Here's how the part is built. I have some questions about the finished solid (model axes, mm). A direction names the side the tool comes from. Coordinates: 2 decimals unless noted, no trailing zeros. Write each loop counter-clockwise with the first axis right and the second up, starting at its lowest first coordinate (ties: lowest second). Pieces come first, ordered by that corner, then holes. Notation, with made-up numbers: (0, -17) -> (40, -17) arc R4 cw to (40, -13) -> close; hole circle Ø1 at (-2, 61.25). An arc over 180 degrees is marked (long way). Use a Markdown table: item, result. Add a question column.
```python
from build123d import *

# Parameters (mm, degrees)
SKETCH1_W           = 50
SKETCH1_H           = 50
BOSS_EXTRUDE1_DEPTH = 10
SKETCH2_R           = 17
CUT_EXTRUDE1_DEPTH  = 10
SKETCH3_R           = 4
BOSS_EXTRUDE2_DEPTH = 10


with BuildPart() as part:
    # Sketch1 → Boss-Extrude1 (new body)
    with BuildSketch(Plane.XY):
        Rectangle(SKETCH1_W, SKETCH1_H)
    extrude(amount=BOSS_EXTRUDE1_DEPTH)

    # Sketch2 → Cut-Extrude1 (cut)
    with BuildSketch(Plane.XY.offset(10)):
        Circle(SKETCH2_R)
    extrude(amount=-CUT_EXTRUDE1_DEPTH, mode=Mode.SUBTRACT)

    # Sketch3 → Boss-Extrude2 (add)
    with BuildSketch(Plane(origin=(0, 25, 0), x_dir=(1, 0, 0), z_dir=(0, 1, 0))):
        with Locations(Location((0, -5, 0), (0, 0, 270))):
            Circle(SKETCH3_R)
    boss_extrude2 = extrude(amount=BOSS_EXTRUDE2_DEPTH)

    # Mirror1: Boss-Extrude2 across plane
    add(boss_extrude2.mirror(Plane.ZX))


solid = part.part
```
Q1. Thinking about a two-plate mould opening in Y: for faces 1 (the cylindrical face through (9.139, 14.334, 5.07)), 2 (the flat face through (-0.3, 25, 0.5)), 3 (the flat face through (-0.3, -25, 0.5)), 4 (the flat face through (-6, 17, 0)), which applies, released by +Y, released by -Y, zero draft, split by the parting line, or undercut?
Q2. Please list where these lines run through material, in increasing order: line 1 (Y direction, x = 0, z = 2.5); line 2 (Y direction, x = 14, z = 5.5); line 3 (X direction, y = 13.5, z = 3.25).
Q3. Suppose I cut it at A-A, the plane y = 0. Write out the boundary of the cut face in (x, z).
Q4. Suppose I cut it at D-D, the plane x = -7. Write out the boundary of the cut face in (y, z), and give its area (3 significant figures).
Q5. Which directions (+Z, -Z, +X, -X, +Y, -Y) give clear straight access to the entire face, cutting with the end or side of a thin tool? Please do faces 5 (the cylindrical face through (-3.905, -29.93, 4.133)), 6 (the cylindrical face through (-3.905, 29.93, 4.133)), 7 (the flat face through (-6, 17, 10)).
Q6. Suppose I cut it at C-C, the plane z = 5. Write out the boundary of the cut face in (x, y), and give its area (3 significant figures).
Q7. Will these pins go through, and if not, where does the flat tip stop? pin 1 (4 mm diameter, centred on x = 12.5, y = 6.5, fed in from +Z); pin 2 (3 mm diameter, centred on x = 13, z = 7.5, fed in from -Y); pin 3 (5 mm diameter, centred on x = 11.5, z = 2.5, fed in from +Y).
Q8. Suppose I cut it at B-B, the plane x = 0. Write out the boundary of the cut face in (y, z), and give its area (3 significant figures).
Answer key:
| question | item | result |
|---|---|---|
| 1 | face 1 | undercut |
| 1 | face 2 | released by +Y |
| 1 | face 3 | released by -Y |
| 1 | face 4 | zero draft |
| 2 | line 1 | y = -35 to -17, 17 to 35 |
| 2 | line 2 | y = -25 to -9.64, 9.64 to 25 |
| 2 | line 3 | x = -25 to -10.33, 10.33 to 25 |
| 3 | outline | (-25, 0) -> (-17, 0) -> (-17, 10) -> (-25, 10) -> close; (17, 0) -> (25, 0) -> (25, 10) -> (17, 10) -> close |
| 4 | outline | (-25, 0) -> (-15.49, 0) -> (-15.49, 10) -> (-25, 10) -> close; (15.49, 0) -> (25, 0) -> (25, 10) -> (15.49, 10) -> close |
| 4 | area | 190 mm^2 |
| 5 | face 5 | -Y |
| 5 | face 6 | +Y |
| 5 | face 7 | +Z, +X, -X, +Y, -Y |
| 6 | outline | (-25, -25) -> (-4, -25) -> (-4, -35) -> (4, -35) -> (4, -25) -> (25, -25) -> (25, 25) -> (4, 25) -> (4, 35) -> (-4, 35) -> (-4, 25) -> (-25, 25) -> close; hole circle Ø34 at (0, 0) |
| 6 | area | 1,750 mm^2 |
| 7 | pin 1 | passes through |
| 7 | pin 2 | stops at y = -25 |
| 7 | pin 3 | stops at y = 25 |
| 8 | outline | (-35, 1) -> (-25, 1) -> (-25, 0) -> (-17, 0) -> (-17, 10) -> (-25, 10) -> (-25, 9) -> (-35, 9) -> close; (17, 0) -> (25, 0) -> (25, 1) -> (35, 1) -> (35, 9) -> (25, 9) -> (25, 10) -> (17, 10) -> close |
| 8 | area | 320 mm^2 |
